from build123d import *

# Parameters (mm, degrees)
SKETCH2_R            = 4.525
BOSS_EXTRUDE1_DEPTH  = 1.5
M3_CLEARANCE_HOLE1_D = 3.4
FILLET1_R            = 1


with BuildPart() as part:
    # Sketch2 → Boss-Extrude1 (new body)
    with BuildSketch(Plane(origin=(0, 0, 0), x_dir=(1, 0, 0), z_dir=(0, 1, 0))):
        with Locations((0, -29)):
            Circle(SKETCH2_R)
        with BuildLine():
            Line((3.199658185, -25.800341815), (3.199658185, 25.800341815))
            ThreePointArc((3.199658185, 25.800341815), (0, 24.475), (-3.199658185, 25.800341815))
            Line((-3.199658185, 25.800341815), (-3.199658185, -25.800341815))
            ThreePointArc((-3.199658185, -25.800341815), (0, -24.475), (3.199658185, -25.800341815))
        make_face()
        with Locations((0, 29)):
            Circle(SKETCH2_R)
    extrude(amount=BOSS_EXTRUDE1_DEPTH)

    # M3 Clearance Hole1 (through all)
    with Locations(Plane(origin=(0, 1.5, 0), x_dir=(1, 0, 0), z_dir=(0, 1, 0))):
        with Locations((0, 29), (0, -29)):
            Hole(M3_CLEARANCE_HOLE1_D / 2)

    # Fillet1
    fillet1_edges = [part.edges().sort_by_distance(p)[0] for p in [
        (-3.199658185, 0.75, 25.800341815),
        (-3.199658185, 0.75, -25.800341815),
        (3.199658185, 0.75, -25.800341815),
        (3.199658185, 0.75, 25.800341815),
    ]]
    fillet(fillet1_edges, radius=FILLET1_R)


solid = part.part
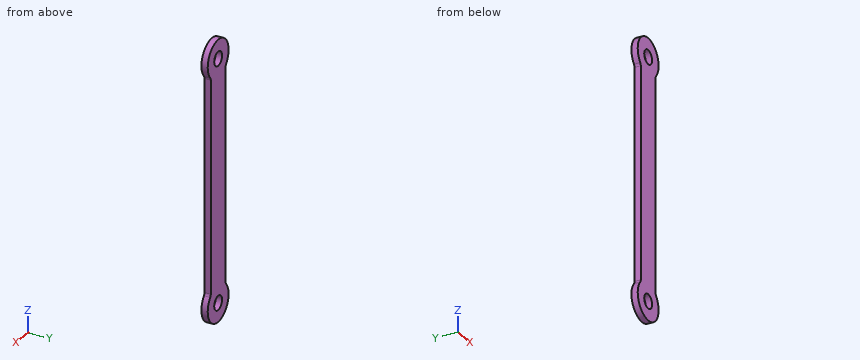
The listing builds one solid part. Answer for the finished solid, in the listing's coordinates (mm). Round coordinates to 2 decimals unless told otherwise and drop trailing zeros. Loops run counter-clockwise (first coordinate to the right, second up) from the corner with the lowest first, then second, coordinate; pieces in that order, holes last. Notation, with made-up numbers: M 50.25,17.25 L 60.25,17.25 A8 ccw 60.25,24.25 Z; hole C 50,-12.5 d5. An arc over 180 degrees is marked long. Return JSON: item names as keys, results as strings.
Q1. Find section D-D, the plane z = 7.5. Determine the outline of the cut face in (x, y).
Results list:
{"outline": "M -3.2,0 L 3.2,0 L 3.2,1.5 L -3.2,1.5 Z"}
Q2. Find section A-A, the plane x = 0. Determine the outline of the cut face in (y, z) (3 decimals), plus the area to 3 significant figures.
Results list:
{"outline": "M 0,-33.525 L 1.5,-33.525 L 1.5,-30.7 L 0,-30.7 Z; M 0,-27.3 L 1.5,-27.3 L 1.5,27.3 L 0,27.3 Z; M 0,30.7 L 1.5,30.7 L 1.5,33.525 L 0,33.525 Z", "area": "90.4 mm2"}
Q3. Find section C-C, the plane y = 1.2. Determine the outline of the cut face in (x, z) (3 decimals).
Results list:
{"outline": "M -3.44,-26.06 A4.525 ccw long 3.44,-26.06 A1 cw 3.2,-25.41 L 3.2,25.41 A1 cw 3.44,26.06 A4.525 ccw long -3.44,26.06 A1 cw -3.2,25.41 L -3.2,-25.41 A1 cw Z; hole C 0,-29 d3.4; hole C 0,29 d3.4"}
Q4. Find the intervals of material crossed by line 1 along X through (y, z) = (0.6, 29) (3 decimals); line 2 along Z through (x, y) = (-0.25, 0.35); line 3 along Z through (x, y) = (-0.75, 0.85), in increasing order. Write a range as from..to.
Results list:
{"line 1": "x = -4.525..-1.7, 1.7..4.525", "line 2": "z = -33.52..-30.68, -27.32..27.32, 30.68..33.52", "line 3": "z = -33.46..-30.53, -27.47..27.47, 30.53..33.46"}
Q5. Find section B-B, the plane z = 29. Determine the outline of the cut face in (x, y) (3 decimals).
Results list:
{"outline": "M -4.525,0 L -1.7,0 L -1.7,1.5 L -4.525,1.5 Z; M 1.7,0 L 4.525,0 L 4.525,1.5 L 1.7,1.5 Z"}
